```python
from build123d import *

# Parameters (mm, degrees)
BOSS_EXTRUDE2_DEPTH  = 100
SKETCH2_R            = 12
CUT_EXTRUDE2_DEPTH   = 100
BOSS_EXTRUDE3_DEPTH  = 12
SKETCH4_R            = 24
SKETCH4_R_2          = 12
BOSS_EXTRUDE4_DEPTH  = 34
SKETCH9_W            = 12
SKETCH9_H            = 56.23521347
BOSS_EXTRUDE14_DEPTH = 53
BOSS_EXTRUDE15_DEPTH = 100
CUT_EXTRUDE5_DEPTH   = 100
SKETCH18_W           = 10.631018499
SKETCH18_H           = 16.963963476
CUT_EXTRUDE6_DEPTH   = 2


with BuildPart() as part:
    # Sketch1 → Boss-Extrude2 (new body)
    with BuildSketch(Plane.XY):
        with BuildLine():
            Line((0, 0), (-60, 0))
            Line((-60, 0), (-60, 12))
            Line((-60, 12), (-7.046781234, 12))
            ThreePointArc((-7.046781234, 12), (22.318707009, 27.175300716), (51.684195251, 12))
            Line((51.684195251, 12), (104.637414017, 12))
            Line((104.637414017, 12), (104.637414017, 0))
            Line((104.637414017, 0), (44.637414017, 0))
            ThreePointArc((44.637414017, 0), (22.318707009, 15.175300716), (0, 0))
        make_face()
    extrude(amount=BOSS_EXTRUDE2_DEPTH)

    # Sketch2 → Cut-Extrude2 (cut)
    with BuildSketch(Plane(origin=(0, 0, 0), x_dir=(1, 0, 0), z_dir=(0, 1, 0))):
        with Locations((-33.523390617, -50)):
            Circle(SKETCH2_R)
        with Locations((74.637414017, -50)):
            Circle(SKETCH2_R)
    extrude(amount=CUT_EXTRUDE2_DEPTH, mode=Mode.SUBTRACT)

    # Sketch3 → Boss-Extrude3 (add)
    with BuildSketch(Plane(origin=(0, 0, 0), x_dir=(1, 0, 0), z_dir=(0, 1, 0))):
        with BuildLine():
            Line((-60, 0), (-60, -100))
            ThreePointArc((-60, -100), (-90.100867093, -50), (-60, 0))
        make_face()
        with BuildLine():
            Line((104.637414017, 0), (104.637414017, -100))
            ThreePointArc((104.637414017, -100), (132.946932966, -50), (104.637414017, 0))
        make_face()
    extrude(amount=BOSS_EXTRUDE3_DEPTH)



with BuildPart() as body_2:
    # Sketch4 → Boss-Extrude4 (new body)
    with BuildSketch(Plane.XY):
        with Locations((22.318707009, 79.175300716)):
            Circle(SKETCH4_R)
        with Locations((22.318707009, 79.175300716)):
            Circle(SKETCH4_R_2, mode=Mode.SUBTRACT)
    extrude(amount=BOSS_EXTRUDE4_DEPTH)


with BuildPart() as part_1:
    add(part.part)

    add(body_2.part)  # Boss-Extrude14 merges body 2
    # Sketch9 → Boss-Extrude14 (add)
    with BuildSketch(Plane.ZY.offset(1.681292991)):
        with Locations((6, 40.117606735)):
            Rectangle(SKETCH9_W, SKETCH9_H)
    extrude(amount=-BOSS_EXTRUDE14_DEPTH)

    # Sketch15 → Boss-Extrude15 (add)
    with BuildSketch(Plane.XY):
        Polygon((15.430799057, 55.991491628), (15.430799057, 26.510222876), (29.20661496, 26.510222876), (28.524429867, 55.991491628), align=None)
    extrude(amount=BOSS_EXTRUDE15_DEPTH)

    # Sketch16 → Cut-Extrude5 (cut)
    with BuildSketch(Plane(origin=(29.804092856, 0.689655118, 0), x_dir=(0, 0, -1), z_dir=(0.999732387, 0.023133419, 0))):
        Polygon((-34, 55.316639981), (-100, 25.827479536), (-100, 55.316639981), (-101.715628872, 69.701769469), (-35.158701994, 67.524066269), align=None)
    extrude(amount=-CUT_EXTRUDE5_DEPTH, mode=Mode.SUBTRACT)

    # Sketch18 → Cut-Extrude6 (cut)
    with BuildSketch(Plane(origin=(0, 68.23521347, 0), x_dir=(1, 0, 0), z_dir=(0, 1, 0))):
        with Locations((22.703243631, -8.481981738)):
            Rectangle(SKETCH18_W, SKETCH18_H)
    extrude(amount=-CUT_EXTRUDE6_DEPTH, mode=Mode.SUBTRACT)


solid = part_1.part
```
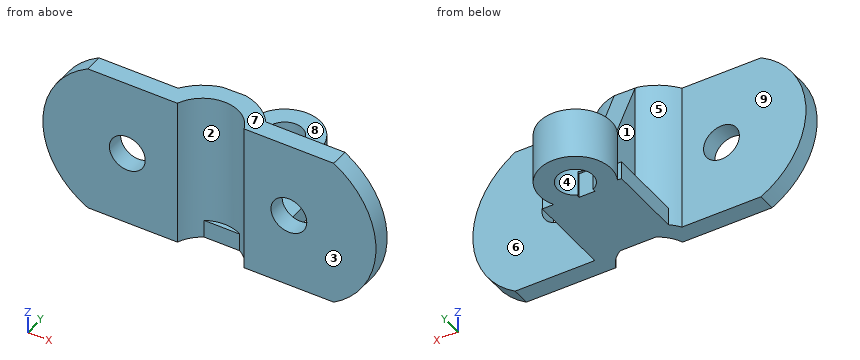
Design review of the part built by this model. Coordinates are the model's own, in mm. Face numbers are marked on the shaded views. A direction names the side the tool comes from. Give positions to 0.01 mm unless a question says otherwise; leave off trailing zeros. Order: outer loops, then holes, each group sorted by start corner. A loop starts at its lowest first (then second) coordinate and runs counter-clockwise, first axis right, second up. Notation, with made-up numbers: (-23, 50.25) -> (-17, 50.25) arc R30 cw to (-17, 85.25) -> close; hole circle Ø1 at (17, 88.5). An arc over 180 degrees is marked (long way). Write item = value, one per line. Start each with the question number.
(1) For pin 1 (1.6 mm diameter, centred on x = 23, y = 13, fed in from +Z); pin 2 (2 mm diameter, centred on x = 34, z = 72, fed in from +Y); pin 3 (3.5 mm diameter, centred on y = 47.5, z = 4.5, fed in from -X), all flat-tipped, find the tip position at first contact; note any pin that passes through.
(2) We need section B-B on x = -29. Write out the cut boundary in (y, z), plus the area to 3 significant figures.
(3) To check wall thickness, follow line 1 along Y through (x, z) = (23, 13); line 2 along X through (y, z) = (2.75, 50); line 3 along Z through (x, y) = (12.5, 64). State the ranges of each line that lie inside material, in increasing order.
(4) We need section A-A on z = 54. Write out the cut boundary in (x, y), plus the area to 3 significant figures.
(5) Mouldability with a two-part tool opening along X and no side actions: class the marked faces 1, 2, 3 and 4 as +X half, -X half, draft (parallel to the pull), parting line (faces both ways), or undercut.
(6) For the marked faces 5, 6, 7, 8 and 9, list the 3-axis set-ups (+Z, -Z, +X, -X, +Y, -Y) from which the entire face can be reached by the end or side of a thin tool; tool diameter is ignored.
(7) We need section D-D on y = 30.5. Write out the cut boundary in (x, z), plus the area to 3 significant figures.
(8) We need section C-C on y = 74. Write out the cut boundary in (x, z).
Numbers:
q1.pin_1 = 12
q1.pin_2 = 25.55
q1.pin_3 = -1.68
q2.outline = (0, 0) -> (12, 0) -> (12, 38.89) -> (0, 38.89) -> close; (0, 61.11) -> (12, 61.11) -> (12, 100) -> (0, 100) -> close
q2.area = 933 mm^2
q3.line_1 = 15.17 to 66.24, 91.16 to 103.17
q3.line_2 = -90.1 to -45.52, -21.52 to 1.29, 43.34 to 62.64, 86.64 to 132.95
q3.line_3 = 0 to 34
q4.outline = (-89.96, 0) -> (-44.84, 0) -> (-44.84, 12) -> (-89.96, 12) -> close; (-22.21, 0) -> (0, 0) arc R24 cw to (44.64, 0) -> (63.32, 0) -> (63.32, 12) -> (51.68, 12) arc R36 ccw to (29.21, 26.51) -> (28.73, 47.06) -> (15.43, 46.75) -> (15.43, 26.51) arc R36 ccw to (-7.05, 12) -> (-22.21, 12) -> close; (85.95, 0) -> (132.81, 0) -> (132.81, 12) -> (85.95, 12) -> close
q4.area = 2,530 mm^2
q5.face_1 = -X half
q5.face_2 = undercut
q5.face_3 = draft
q5.face_4 = undercut
q6.face_5 = +Z, -X
q6.face_6 = +Z, -Z, +X, +Y
q6.face_7 = +Z, +X, -X, +Y, -Y
q6.face_8 = +Z, +X, -X, +Y
q6.face_9 = +Z, -Z, -X, +Y
q7.outline = (-1.68, 0) -> (51.32, 0) -> (51.32, 12) -> (29.11, 12) -> (29.11, 91.07) -> (15.43, 90.36) -> (15.43, 12) -> (-1.68, 12) -> close
q7.area = 1,710 mm^2
q8.outline = (-1.12, 0) -> (11.49, 0) -> (11.49, 34) -> (-1.12, 34) -> close; (33.15, 0) -> (45.75, 0) -> (45.75, 34) -> (33.15, 34) -> close
